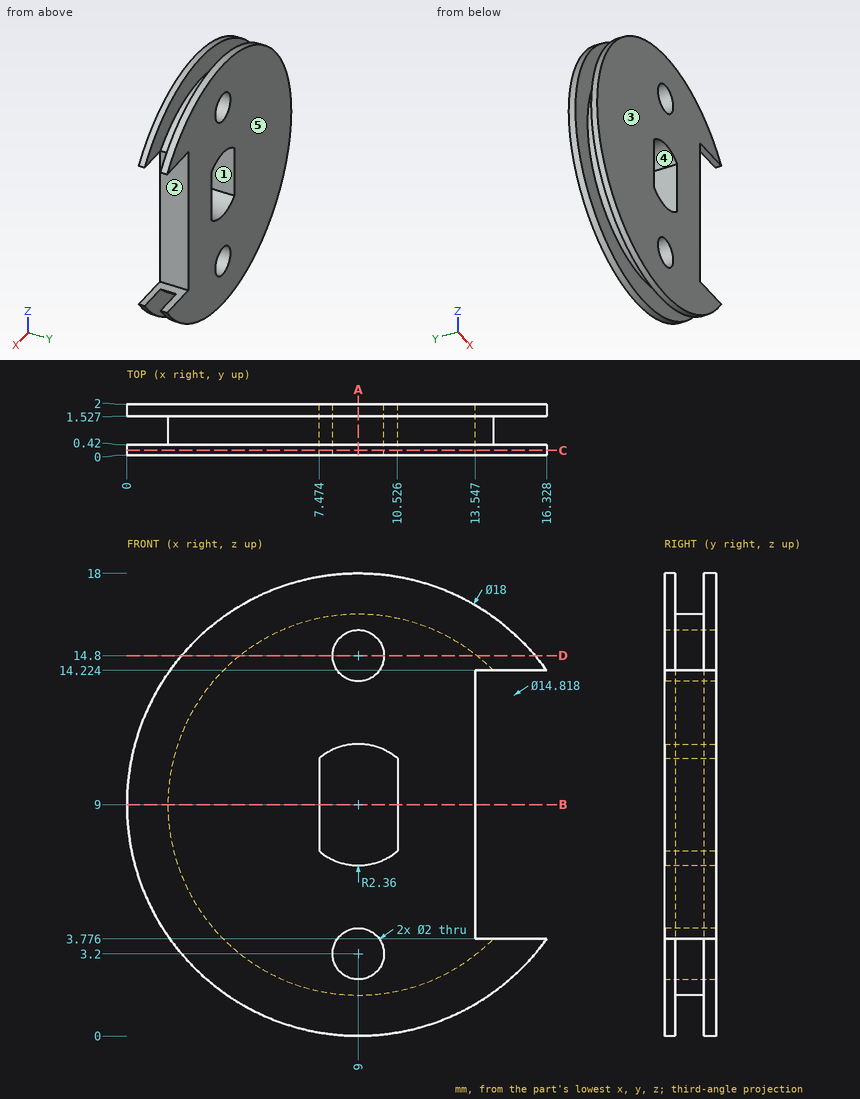
Source: three-view drawing plus pictorial views. Frame: mm from the lowest corner of the part. A direction names the side the tool comes from. Round coordinates to 2 decimals unless told otherwise and drop trailing zeros. Order: outer loops, then holes, each group sorted by start corner. A loop starts at its lowest first (then second) coordinate and runs counter-clockwise, first axis right, second up. Notation, with made-up numbers: (55, -33.5) - (72, -33.5) arc R15 cw to (72, -16.5) - close; hole circle Ø7 at (14.5, -22.5). An arc over 180 degrees is marked (long way). Use a Markdown table: item, result.
1. Access query for the marked faces 1, 2 and 3. Directions: +Z, -Z, +X, -X, +Y, -Y. A direction counts if a zero-diameter tool reaches every point of the face in a straight line with its end or side. Return the directions, or none.
Evaluation:
| item | result |
|---|---|
| face 1 | +Y, -Y |
| face 2 | +X, +Y, -Y |
| face 3 | +Z, -Z, +X, -X, -Y |
2. Section A-A on x = 9. Return the cut outline in (y, z).
Evaluation:
| item | result |
|---|---|
| outline | (0, 0) - (0.42, 0) - (0.42, 1.59) - (1.53, 1.59) - (1.53, 0) - (2, 0) - (2, 2.2) - (0, 2.2) - close; (0, 4.2) - (2, 4.2) - (2, 6.64) - (0, 6.64) - close; (0, 11.36) - (2, 11.36) - (2, 13.8) - (0, 13.8) - close; (0, 15.8) - (2, 15.8) - (2, 18) - (1.53, 18) - (1.53, 16.41) - (0.42, 16.41) - (0.42, 18) - (0, 18) - close |
3. Material intervals for probe 1 along Y at (x, z) = (14, 14.75); probe 2 along Z at (x, y) = (9.5, 1.6) (1 decimal); probe 3 along X at (y, z) = (0.6, 8.5), sorted ascending.
Evaluation:
| item | result |
|---|---|
| probe 1 | 0 to 0.42, 1.53 to 2 |
| probe 2 | 0 to 2.3, 4.1 to 6.7, 11.3 to 13.9, 15.7 to 18 |
| probe 3 | 1.61 to 7.47, 10.53 to 13.55 |
4. Section C-C on y = 0.2. Return the cut outline in (x, z) (1 decimal), then the cut area to 3 significant figures.
Evaluation:
| item | result |
|---|---|
| outline | (13.5, 3.8) - (13.5, 14.2) - (16.3, 14.2) arc R9 ccw (long way) to (16.3, 3.8) - close; hole (7.5, 7.2) arc R2.4 ccw to (10.5, 7.2) - (10.5, 10.8) arc R2.4 ccw to (7.5, 10.8) - close; hole circle Ø2 at (9, 3.2); hole circle Ø2 at (9, 14.8) |
| area | 194 mm^2 |
5. First-contact query: pin 1 (1.5 mm diameter, centred on x = 14.5, z = 9, fed in from +Y); pin 2 (0.6 mm diameter, centred on y = 1, z = 9, fed in from +X). Flat tips, straight axial feed; report the tip coordinate or a pass-through.
Evaluation:
| item | result |
|---|---|
| pin 1 | through |
| pin 2 | x = 13.55 |
6. Mould query, pull axis Z, two halves, no side actions, for the marked faces 4 and 5. Classes: +Z half, -Z half, draft (parallel to the pull), parting line (faces both ways), or undercut.
Evaluation:
| item | result |
|---|---|
| face 4 | undercut |
| face 5 | draft |
7. Section D-D on z = 14.8. Return the cut outline in (x, y).
Evaluation:
| item | result |
|---|---|
| outline | (2.12, 0) - (8, 0) - (8, 2) - (2.12, 2) - (2.12, 1.53) - (4.39, 1.53) - (4.39, 0.42) - (2.12, 0.42) - close; (10, 0) - (15.88, 0) - (15.88, 0.42) - (13.61, 0.42) - (13.61, 1.53) - (15.88, 1.53) - (15.88, 2) - (10, 2) - close |
8. Section B-B on z = 9. Return the cut outline in (x, y).
Evaluation:
| item | result |
|---|---|
| outline | (0, 0) - (7.47, 0) - (7.47, 2) - (0, 2) - (0, 1.53) - (1.59, 1.53) - (1.59, 0.42) - (0, 0.42) - close; (10.53, 0) - (13.55, 0) - (13.55, 2) - (10.53, 2) - close |
